Source: CAD feature listing. Evaluate the final solid. Frame: model axes, mm. Give positions to 0.01 mm unless a question says otherwise; leave off trailing zeros. Write each loop counter-clockwise with the first axis right and the second up, starting at its lowest first coordinate (ties: lowest second). Pieces come first, ordered by that corner, then holes.
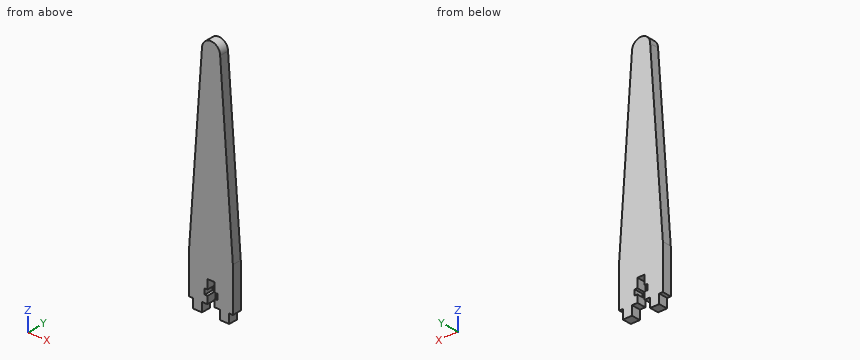
```python
from build123d import *

# Parameters (mm, degrees)
BOSS_EXTRUDE1_DEPTH = 5


with BuildPart() as part:
    # Sketch1 → Boss-Extrude1 (new body)
    with BuildSketch(Plane(origin=(0, 0, 0), x_dir=(1, 0, 0), z_dir=(0, 1, 0))):
        with BuildLine():
            Line((0, 0), (0, 24))
            Line((0, 24), (2, 24))
            Line((2, 24), (2, 29))
            Line((2, 29), (7, 29))
            Line((7, 29), (7, 24))
            Line((7, 24), (10, 24))
            Line((10, 24), (10, 20))
            Line((10, 20), (8.5, 20))
            Line((8.5, 20), (8.5, 17))
            Line((8.5, 17), (10, 17))
            Line((10, 17), (10, 12))
            Line((10, 12), (14, 12))
            Line((14, 12), (14, 17))
            Line((14, 17), (15.5, 17))
            Line((15.5, 17), (15.5, 20))
            Line((15.5, 20), (14, 20))
            Line((14, 20), (14, 24))
            Line((14, 24), (17, 24))
            Line((17, 24), (17, 29))
            Line((17, 29), (22, 29))
            Line((22, 29), (22, 24))
            Line((22, 24), (24, 24))
            Line((24, 24), (24, 0))
            Line((24, 0), (17, -97))
            ThreePointArc((17, -97), (12, -102), (7, -97))
            Line((7, -97), (0, 0))
        make_face()
    extrude(amount=BOSS_EXTRUDE1_DEPTH)


solid = part.part
```
1. Section query C-C (z = 68.5). Return loops of the section in (x, y), plus the area to 3 significant figures.
2. Section query B-B (x = 12). Return loops of the section in (y, z).
3. Pin query (flat end, axial travel): P1, Ø1.6, axis at x = 14.5, y = 3, coming from the +Z side; P2, Ø2, axis at y = 3, z = 34, coming from the -X side; P3, Ø1.6, axis at x = 9, y = 1.5, coming from the +Z side. Return the tip coordinate at first contact, or that it passes through.
4. Line query: probe 1 along X at (y, z) = (2.6, -19); probe 2 along X at (y, z) = (1.3, -23); probe 3 along Z at (x, y) = (15, 2.8). Output: solid intervals per line, ascending.
5. Section query A-A (y = 1.1). Return loops of the section in (x, z), plus the area to 3 significant figures.
The answers:
1. outline: (4.94, 0) - (19.06, 0) - (19.06, 5) - (4.94, 5) - close
1. area: 70.6 mm2
2. outline: (0, -12) - (5, -12) - (5, 102) - (0, 102) - close
3. P1: stops at z = 101.7
3. P2: stops at x = 2.38
3. P3: stops at z = 101.49
4. probe 1: x = 0 to 8.5, 15.5 to 24
4. probe 2: x = 0 to 10, 14 to 24
4. probe 3: z = -24 to -20, -17 to 101
5. outline: (0, -24) - (2, -24) - (2, -29) - (7, -29) - (7, -24) - (10, -24) - (10, -20) - (8.5, -20) - (8.5, -17) - (10, -17) - (10, -12) - (14, -12) - (14, -17) - (15.5, -17) - (15.5, -20) - (14, -20) - (14, -24) - (17, -24) - (17, -29) - (22, -29) - (22, -24) - (24, -24) - (24, 0) - (17, 97) arc R5 ccw to (7, 97) - (0, 0) - close
5. area: 2,260 mm2
